from build123d import *

# Parameters (mm, degrees)
SKETCH_W        = 65
SKETCH_H        = 160
PAD_DEPTH       = 10
POCKET_DEPTH    = 7
SKETCH003_R     = 1.6
POCKET002_DEPTH = 10
POCKET003_DEPTH = 10
SKETCH005_R     = 1.6
POCKET004_DEPTH = 10
SKETCH006_R     = 1.6
POCKET005_DEPTH = 10
SKETCH007_W     = 5.7
SKETCH007_H     = 2.6
POCKET006_DEPTH = 6.15
POCKET007_DEPTH = 11
SKETCH010_R     = 4
SKETCH010_R_2   = 1.6
POCKET008_DEPTH = 10
POCKET009_DEPTH = 2.7


with BuildPart() as part:
    # Sketch → Pad (new body)
    with BuildSketch(Plane.XY):
        with Locations((32.5, 80)):
            Rectangle(SKETCH_W, SKETCH_H)
    extrude(amount=PAD_DEPTH)

    # Sketch001 (on Face6 of Pad) → Pocket (cut)
    with BuildSketch(Plane.XY.offset(10)):
        Polygon((24.9, 6.1), (40.1, 6.1), (37.6, 0), (27.4, 0), align=None)
        Polygon((49.9, 6.1), (65.1, 6.1), (62.6, 0), (52.4, 0), align=None)
        Polygon((-0.1, 6.1), (15.1, 6.1), (12.6, 0), (2.4, 0), align=None)
        Polygon((39.7, 153.9), (24.9, 153.9), (27.4, 160), (37.2, 160), align=None)
        Polygon((14.7, 153.9), (-0.1, 153.9), (2.4, 160), (12.2, 160), align=None)
        Polygon((64.7, 153.9), (49.9, 153.9), (52.4, 160), (62.2, 160), align=None)
    extrude(amount=-POCKET_DEPTH, mode=Mode.SUBTRACT)

    # Sketch003 → Pocket002 (cut)
    with BuildSketch(Plane.XY.offset(10)):
        with Locations((20, 157)):
            Circle(SKETCH003_R)
        with Locations((45, 157)):
            Circle(SKETCH003_R)
        with Locations((20, 3)):
            Circle(SKETCH003_R)
        with Locations((45, 3)):
            Circle(SKETCH003_R)
    extrude(amount=-POCKET002_DEPTH, mode=Mode.SUBTRACT)

    # Sketch004 (on Face2 of Pocket002) → Pocket003 (cut)
    with BuildSketch(Plane(origin=(0, 0, 0), x_dir=(1, 0, 0), z_dir=(0, 0, -1))):
        Polygon((58.9, -84.9), (58.9, -100.1), (65, -97.6), (65, -87.4), align=None)
        Polygon((58.9, -59.9), (58.9, -75.1), (65, -72.6), (65, -62.4), align=None)
        Polygon((58.9, -34.9), (58.9, -50.1), (65, -47.6), (65, -37.4), align=None)
        Polygon((58.9, -9.9), (58.9, -25.1), (65, -22.6), (65, -12.4), align=None)
        Polygon((58.9, -134.9), (58.9, -150.1), (65, -147.6), (65, -137.4), align=None)
        Polygon((58.9, -109.9), (58.9, -125.1), (65, -122.6), (65, -112.4), align=None)
        Polygon((0, -14.9), (0, -25.1), (6.1, -27.6), (6.1, -12.4), align=None)
        Polygon((0, -39.9), (0, -50.1), (6.1, -52.6), (6.1, -37.4), align=None)
        Polygon((0, -64.9), (0, -75.1), (6.1, -77.6), (6.1, -62.4), align=None)
        Polygon((0, -89.9), (0, -100.1), (6.1, -102.6), (6.1, -87.4), align=None)
        Polygon((0, -114.9), (0, -125.1), (6.1, -127.6), (6.1, -112.4), align=None)
        Polygon((0, -139.9), (0, -150.1), (6.1, -152.6), (6.1, -137.4), align=None)
    extrude(amount=-POCKET003_DEPTH, mode=Mode.SUBTRACT)

    # Sketch005 (on Face40 of Pocket003) → Pocket004 (cut)
    with BuildSketch(Plane.XZ):
        with Locations((20, 7)):
            Circle(SKETCH005_R)
        with Locations((45, 7)):
            Circle(SKETCH005_R)
    extrude(amount=-POCKET004_DEPTH, mode=Mode.SUBTRACT)

    # Sketch006 (on Face1 of Pocket004) → Pocket005 (cut)
    with BuildSketch(Plane(origin=(0, 160, 0), x_dir=(-1, 0, 0), z_dir=(0, 1, 0))):
        with Locations((-45, 7)):
            Circle(SKETCH006_R)
        with Locations((-20, 7)):
            Circle(SKETCH006_R)
    extrude(amount=-POCKET005_DEPTH, mode=Mode.SUBTRACT)

    # Sketch007 (on Face6 of Pocket005) → Pocket006 (cut)
    with BuildSketch(Plane.XY.offset(10)):
        with Locations((20, 157)):
            Rectangle(SKETCH007_W, SKETCH007_H)
        with Locations((45, 157)):
            Rectangle(SKETCH007_W, SKETCH007_H)
        with Locations((20, 3)):
            Rectangle(SKETCH007_W, SKETCH007_H)
        with Locations((45, 3)):
            Rectangle(SKETCH007_W, SKETCH007_H)
    extrude(amount=-POCKET006_DEPTH, mode=Mode.SUBTRACT)

    # Sketch009 (on Face6 of Pocket006) → Pocket007 (cut)
    with BuildSketch(Plane.XY.offset(10)):
        Polygon((14.9, 113.6), (25.1, 113.6), (27.6, 107.5), (12.4, 107.5), align=None)
        Polygon((39.9, 113.6), (50.1, 113.6), (52.6, 107.5), (37.4, 107.5), align=None)
        Polygon((12.4, 52.5), (27.6, 52.5), (25.1, 46.4), (14.9, 46.4), align=None)
        Polygon((37.4, 52.5), (52.6, 52.5), (50.1, 46.4), (39.9, 46.4), align=None)
    extrude(amount=-POCKET007_DEPTH, mode=Mode.SUBTRACT)

    # Sketch010 (on Face6 of Pocket007) → Pocket008 (cut)
    with BuildSketch(Plane.XY.offset(10)):
        with Locations((32.5, 80)):
            Circle(SKETCH010_R)
        with Locations((32.5, 95)):
            Circle(SKETCH010_R_2)
        with Locations((32.5, 65)):
            Circle(SKETCH010_R_2)
    extrude(amount=-POCKET008_DEPTH, mode=Mode.SUBTRACT)

    # Sketch011 (on Face6 of Pocket008) → Pocket009 (cut)
    with BuildSketch(Plane.XY.offset(10)):
        Polygon((35.275, 93.397853), (35.275, 96.602147), (32.5, 98.204294), (29.725, 96.602147), (29.725, 93.397853), (32.5, 91.795706), align=None)
        Polygon((35.275, 63.397853), (35.275, 66.602147), (32.5, 68.204294), (29.725, 66.602147), (29.725, 63.397853), (32.5, 61.795706), align=None)
    extrude(amount=-POCKET009_DEPTH, mode=Mode.SUBTRACT)


solid = part.part
Could you check a few things on this model? Use its own coordinates, in mm. A direction names the side the tool comes from. Round coordinates to 2 decimals unless told otherwise and drop trailing zeros. Order: outer loops, then holes, each group sorted by start corner. A loop starts at its lowest first (then second) coordinate and runs counter-clockwise, first axis right, second up.
(1) Please list where these lines run through material, in increasing order: line 1 along Y through (x, z) = (23, 8.75); line 2 along Y through (x, z) = (47.5, 9.25); line 3 along X through (y, z) = (0.45, 7).
Response values:
line 1: y = 0 to 46.4, 52.5 to 107.5, 113.6 to 160
line 2: y = 0 to 1.7, 4.3 to 46.4, 52.5 to 107.5, 113.6 to 155.7, 158.3 to 160
line 3: x = 0 to 2.22, 12.78 to 18.4, 21.6 to 27.22, 37.78 to 43.4, 46.6 to 52.22, 62.78 to 65
(2) Which directions (+Z, -Z, +X, -X, +Y, -Y) give clear straight access to the entire face, cutting with the end or side of a thin tool? Please do faces 1 (the flat face through (25, 81, 0)), 2 (the flat face through (6.1, 120, 5)), 3 (the flat face through (31.09, 62.61, 8.67)).
Response values:
face 1: -Z, +X, -X, +Y, -Y
face 2: +Z, -Z
face 3: +Z
(3) I'm going to push flat-ended pins straight in: pin 1 (0.8 mm diameter, centred on y = 64.5, z = 8.5, fed in from +X); pin 2 (1 mm diameter, centred on x = 19.5, z = 7, fed in from +Y); pin 3 (2 mm diameter, centred on x = 57.5, z = 8, fed in from -Y). Where does each tip first touch, or does it pass through?
Response values:
pin 1: stops at x = 58.9
pin 2: stops at y = 150
pin 3: stops at y = 6.1
(4) Imagine slicing it at B-B (z = 1.5). Count the separate pieces of the cut face and the enclosed holes in it, plus the area to 3 significant figures.
Response values:
separate pieces: 1
enclosed holes: 11
area: 9,060 mm2
(5) Imagine slicing it at A-A (y = 95). Write out the boundary of the cut face in (x, z) (3 decimals), plus the area to 3 significant figures.
Response values:
outline: (6.1, 0) - (30.9, 0) - (30.9, 7.3) - (29.725, 7.3) - (29.725, 10) - (6.1, 10) - close; (34.1, 0) - (58.9, 0) - (58.9, 10) - (35.275, 10) - (35.275, 7.3) - (34.1, 7.3) - close
area: 490 mm2
(6) If we mould it in two halves opening along X, with no side actions, what happens to faces 4 (the flat face through (65, 130, 5)), 5 (the flat face through (32, 160, 2.7)), 6 (the flat face through (0, 57, 5)), 7 (the flat face through (61.993, 86.168, 4.93))? For each: released by +X, released by -X, zero draft, split by the parting line, or undercut.
Response values:
face 4: released by +X
face 5: zero draft
face 6: released by -X
face 7: undercut
(7) Imagine slicing it at C-C (x = 56). Write out the boundary of the cut face in (y, z), plus the area to 3 significant figures.
Response values:
outline: (0, 0) - (160, 0) - (160, 3) - (153.9, 3) - (153.9, 10) - (6.1, 10) - (6.1, 3) - (0, 3) - close
area: 1,510 mm2
